```python
from build123d import *

# Parameters (mm, degrees)
SKETCH_1_R      = 2.25
SKETCH_1_R_2    = 1.7
SKETCH_1_R_3    = 5
SKETCH_1_R_4    = 1.69491354
EXTRUDE_1_DEPTH = 4


with BuildPart() as part:
    # 草图1 → 凸台-拉伸1 (new body)
    with BuildSketch(Plane(origin=(0, 0, 0), x_dir=(1, 0, 0), z_dir=(0, 1, 0))):
        Polygon((44.23849367, 33.250010702), (44.23849367, 25.250010702), (26.23849367, 12), (26.23849367, -12), (44.23849367, -25.250010702), (44.23849367, -31.250010702), (29.23849367, -46.250010702), (26.23849367, -46.250010702), (17, -30.248470281), (-17, -30.248470281), (-26.23849367, -46.250010702), (-34.23849367, -46.250010702), (-44.23849367, -36.250010702), (-44.23849367, -25.250010702), (-26.23849367, -12), (-26.23849367, 12), (-44.23849367, 25.250010702), (-44.23849367, 33.250010702), (-31.23849367, 46.250010702), (-26.23849367, 46.250010702), (-17, 30.248470281), (17, 30.248470281), (26.23849367, 46.250010702), (31.23849367, 46.250010702), align=None)
        with Locations(Location((-15.25, -15.25, 0), (0, 0, 270))):
            Circle(SKETCH_1_R, mode=Mode.SUBTRACT)
        with Locations(Location((-15.25, 15.25, 0), (0, 0, 270))):
            Circle(SKETCH_1_R, mode=Mode.SUBTRACT)
        with Locations(Location((15.25, -15.25, 0), (0, 0, 270))):
            Circle(SKETCH_1_R, mode=Mode.SUBTRACT)
        with Locations(Location((15.25, 15.25, 0), (0, 0, 270))):
            Circle(SKETCH_1_R, mode=Mode.SUBTRACT)
        with Locations(Location((-24, -33, 0), (0, 0, 270))):
            Circle(SKETCH_1_R_2, mode=Mode.SUBTRACT)
        with Locations(Location((-16, 0, 0), (0, 0, 270))):
            Circle(SKETCH_1_R_3, mode=Mode.SUBTRACT)
        with Locations(Location((0, 24, 0), (0, 0, 270))):
            Circle(SKETCH_1_R_3, mode=Mode.SUBTRACT)
        with Locations(Location((-30.40559154, -40.30508646, 0), (0, 0, 270))):
            Circle(SKETCH_1_R_2, mode=Mode.SUBTRACT)
        with Locations(Location((-30.40559154, 40.30508646, 0), (0, 0, 270))):
            Circle(SKETCH_1_R_2, mode=Mode.SUBTRACT)
        with Locations(Location((-40.30508646, 30.40559154, 0), (0, 0, 270))):
            Circle(SKETCH_1_R_2, mode=Mode.SUBTRACT)
        with Locations(Location((30.40559154, -40.30508646, 0), (0, 0, 270))):
            Circle(SKETCH_1_R_2, mode=Mode.SUBTRACT)
        with Locations(Location((40.30508646, -31, 0), (0, 0, 270))):
            Circle(SKETCH_1_R_4, mode=Mode.SUBTRACT)
        with Locations(Location((40.30508646, 30.40559154, 0), (0, 0, 270))):
            Circle(SKETCH_1_R_4, mode=Mode.SUBTRACT)
        with Locations(Location((30.40559154, 40.30508646, 0), (0, 0, 270))):
            Circle(SKETCH_1_R_2, mode=Mode.SUBTRACT)
        with Locations(Location((-40.30508646, -30.40559154, 0), (0, 0, 90))):
            Circle(SKETCH_1_R_2, mode=Mode.SUBTRACT)
        with Locations(Location((24, -33, 0), (0, 0, 90))):
            Circle(SKETCH_1_R_2, mode=Mode.SUBTRACT)
        with Locations(Location((24, 33, 0), (0, 0, 270))):
            Circle(SKETCH_1_R_2, mode=Mode.SUBTRACT)
        with Locations(Location((-24, 33, 0), (0, 0, 90))):
            Circle(SKETCH_1_R_2, mode=Mode.SUBTRACT)
        with Locations(Location((16, 0, 0), (0, 0, 90))):
            Circle(SKETCH_1_R_3, mode=Mode.SUBTRACT)
        with Locations(Location((0, -24, 0), (0, 0, 90))):
            Circle(SKETCH_1_R_3, mode=Mode.SUBTRACT)
    extrude(amount=EXTRUDE_1_DEPTH)


solid = part.part
```
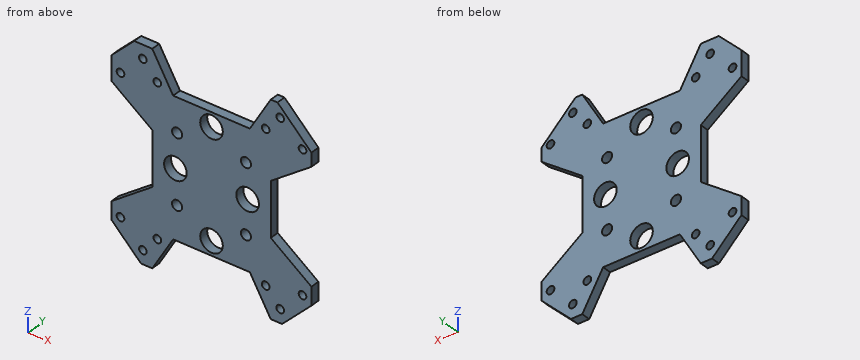
Part model, mm, in its own coordinate system. Round coordinates to 2 decimals unless told otherwise and drop trailing zeros. Order: outer loops, then holes, each group sorted by start corner. A loop starts at its lowest first (then second) coordinate and runs counter-clockwise, first axis right, second up. Notation, with made-up numbers: M -7.5,82 L 51.5,82 A14 ccw 51.5,96 Z; hole C -19,-3.75 d2. An arc over 180 degrees is marked long. Answer in a Markdown table with one row per item. Add a question column.
Q1. Cut at B-B on x = -24. Give the cut face in (y, z).
Q2. Cut at D-D on z = -10. Give the cut face in (x, y), and give its area (3 significant figures).
Q3. Pin check, flat tips, straight feed: pin 1 (1.2 mm diameter, centred on x = -5, y = 1.5, fed in from -Z); pin 2 (4.5 mm diameter, centred on x = -24, z = -33, fed in from -Y); pin 3 (2 mm diameter, centred on y = 2.5, z = -13.5, fed in from -X); pin 4 (2 mm diameter, centred on x = 7, y = 2, fed in from +Z). Stop position of each tip, or through.
Q4. Cut at A-A on z = 15.25. Give the cut face in (x, y), and give its area (3 significant figures).
Q5. Cut at C-C on y = 1.85. Give the number of separate pieces and of enclosed holes in the cut face, and give its area (3 significant figures).
Q6. Wall check: L1, parallel to X at y = 2.35, z = -14.5; L2, parallel to X at y = 3.6, z = -1.5; L3, parallel to Z at x = 31, y = 2.9 (1 decimal). Give the ranges that are in metal, low to high. Write a range as from..to.
Established:
| question | item | result |
|---|---|---|
| 1 | outline | M 0,-42.37 L 4,-42.37 L 4,-34.7 L 0,-34.7 Z; M 0,-31.3 L 4,-31.3 L 4,31.3 L 0,31.3 Z; M 0,34.7 L 4,34.7 L 4,42.37 L 0,42.37 Z |
| 2 | outline | M -26.24,0 L 26.24,0 L 26.24,4 L -26.24,4 Z |
| 2 | area | 210 mm2 |
| 3 | pin 1 | stops at z = -30.25 |
| 3 | pin 2 | stops at y = 0 |
| 3 | pin 3 | stops at x = -29.63 |
| 3 | pin 4 | stops at z = 30.25 |
| 4 | outline | M -30.65,0 L -17.5,0 L -17.5,4 L -30.65,4 Z; M -13,0 L 13,0 L 13,4 L -13,4 Z; M 17.5,0 L 30.65,0 L 30.65,4 L 17.5,4 Z |
| 4 | area | 209 mm2 |
| 5 | separate pieces | 1 |
| 5 | enclosed holes | 20 |
| 5 | area | 4,640 mm2 |
| 6 | L1 | x = -29.63..-17.37, -13.13..13.13, 17.37..29.63 |
| 6 | L2 | x = -26.24..-20.77, -11.23..11.23, 20.77..26.24 |
| 6 | L3 | z = -46.3..-41.9, -38.7..-15.5, 15.5..38.7, 41.9..44.5 |
